from build123d import *

# Parameters (mm, degrees)
F0_W      = 19.05
F0_H      = 19.05
F1_DEPTH  = 19.05
F1_FACE_W = 19.05
F1_FACE_H = 19.05
F2_DEPTH  = 19.05
F3_W      = 19.05
F3_H      = 19.05
F4_DEPTH  = 19.05
F5_W      = 19.05
F5_H      = 19.05
F6_DEPTH  = 19.05
F7_W      = 19.05
F7_H      = 19.05
F8_DEPTH  = 19.05


with BuildPart() as f1:
    # F0 (on Top) → F1 (new body)
    with BuildSketch(Plane.XY):
        with Locations((-9.525, 25.527001)):
            Rectangle(F0_W, F0_H)
    extrude(amount=F1_DEPTH)

    # F1_face (on face) → F2 (join)
    with BuildSketch(Plane(origin=(-9.525, 25.527001, 19.05), x_dir=(1, 0, 0), z_dir=(0, 0, 1))):
        Rectangle(F1_FACE_W, F1_FACE_H)
    extrude(amount=F2_DEPTH)

    # F3 (on face) → F4 (join)
    with BuildSketch(Plane.XZ.offset(-16.002001)):
        with Locations((-9.525, 9.525)):
            Rectangle(F3_W, F3_H)
    extrude(amount=F4_DEPTH)

    # F5 (on face) → F6 (join)
    with BuildSketch(Plane.YZ):
        with Locations((25.527001, 28.575)):
            Rectangle(F5_W, F5_H)
    extrude(amount=F6_DEPTH)

    # F7 (on face) → F8 (join)
    with BuildSketch(Plane(origin=(-19.05, 0, 0), x_dir=(0, -1, 0), z_dir=(-1, 0, 0))):
        with Locations((-25.527001, 28.575)):
            Rectangle(F7_W, F7_H)
    extrude(amount=F8_DEPTH)


solid = f1.part
For this review, take the finished solid that the model builds, in its own axes (mm). A direction names the side the tool comes from. Give positions to 0.01 mm unless a question says otherwise; leave off trailing zeros. Loops run counter-clockwise (first coordinate to the right, second up) from the corner with the lowest first, then second, coordinate; pieces in that order, holes last. Notation, with made-up numbers: (85, 78.5) - (141, 78.5) arc R22 ccw to (141, 102.5) - close; hole circle Ø7 at (51.5, 26.25). An arc over 180 degrees is marked (long way). Write each question's results on one line, items separated by ' | '.
(1) For line 1 along Y through (x, z) = (-20, 20); line 2 along X through (y, z) = (21.5, 3); line 3 along Z through (x, y) = (-23.5, 32), list the stretches that pass through material, from the lowest coordinate up.
Conclusion:
line 1: 16 to 35.05 | line 2: -19.05 to 0 | line 3: 19.05 to 38.1
(2) Take a section at A-A (y = 24). Give the boundary of the cut face in (x, z), then the cut area to 3 significant figures.
Conclusion:
outline: (-38.1, 19.05) - (-19.05, 19.05) - (-19.05, 0) - (0, 0) - (0, 19.05) - (19.05, 19.05) - (19.05, 38.1) - (-38.1, 38.1) - close | area: 1,450 mm^2
(3) For pin 1 Ø6 at (x, y) = (11, 17.5) entering from -Z; pin 2 Ø9.5 at (x, z) = (-6, 26) entering from -Y; pin 3 Ø9.5 at (y, z) = (14.5, 7.5) entering from -X; pin 4 Ø3 at (y, z) = (3.5, 22.5) entering from +X, all flat-tipped, find the tip position at first contact; note any pin that passes through.
Conclusion:
pin 1: z = 19.05 | pin 2: y = 16 | pin 3: x = -19.05 | pin 4: through
(4) Take a section at C-C (x = -27). Give the boundary of the cut face in (y, z), then the cut area to 3 significant figures.
Conclusion:
outline: (16, 19.05) - (35.05, 19.05) - (35.05, 38.1) - (16, 38.1) - close | area: 363 mm^2
(5) Take a section at B-B (z = 29.5). Give the boundary of the cut face in (x, y), then the cut area to 3 significant figures.
Conclusion:
outline: (-38.1, 16) - (19.05, 16) - (19.05, 35.05) - (-38.1, 35.05) - close | area: 1,090 mm^2
(6) For faces 1 (the flat face through (-9, 26, 38.1)), 2 (the flat face through (-28, 26, 19.05)), 3 (the flat face through (-9, 35.052, 23)), 4 (the flat face through (0, 16, 9)), 5 (the flat face through (-9, 16.002, 28)), list the 3-axis set-ups (+Z, -Z, +X, -X, +Y, -Y) from which the entire face can be reached by the end or side of a thin tool; tool diameter is ignored.
Conclusion:
face 1: +Z, +X, -X, +Y, -Y | face 2: -Z, -X, +Y, -Y | face 3: +Z, -Z, +X, -X, +Y | face 4: -Z, +X, +Y, -Y | face 5: +Z, +X, -X, -Y
